Build history of the part. All positions in model axes, mm. A direction names the side the tool comes from. Give positions to 0.01 mm unless a question says otherwise; leave off trailing zeros. Loops run counter-clockwise (first coordinate to the right, second up) from the corner with the lowest first, then second, coordinate; pieces in that order, holes last. Notation, with made-up numbers: (40.25, 53.25) - (68.25, 53.25) arc R11 cw to (68.25, 67.25) - close; hole circle Ø9 at (1.5, 53.25). An arc over 180 degrees is marked (long way). Return JSON: item names as keys, results as strings. Group by question number.
1) 3-axis set-ups, long thin cutter, end or side, ignore diameter. For faces 1 (the face through (-21, 0, -12)), 2 (the face through (-3.365, 1.972, -12.206)): which of +Z, -Z, +X, -X, +Y, -Y reach the whole face in a straight line?
2) Slice it at A-A (x = -4). List the corners of the cut face in (y, z).
3) Mould opens along X. For faces 3 (the face through (-13, 2, 15)), 4 (the face through (5.93, -0.699, 12.785)), 5 (the face through (12, 2, -2)) say: released by +X, released by -X, zero draft, split by the parting line, or undercut.
4) Drop a flat-ended pin along its axis: pin 1 (2 mm diameter, centred on x = 3.5, z = 4, fed in from -Y). Give the stop position or say it passes through.
5) Slice it at D-D (x = -24). List the corners of the cut face in (y, z), and give its area (3 significant figures).
6) Drill centre lines: probe 1 along X at (y, z) = (-0.6, 10); probe 2 along Z at (x, y) = (-4, 1.2); probe 3 along X at (y, z) = (-0.5, -11). Where is each one in solid material? Low to high. Write a range as from..to.
Autodesk Inventor part; units mm, degrees
ref_plane "YZ Plane" through (0, 0, 0) normal (1, 0, 0) x (0, 1, 0)
ref_plane "XZ Plane" through (0, 0, 0) normal (0, 1, 0) x (-1, 0, 0)
ref_plane "XY Plane" through (0, 0, 0) normal (0, 0, 1) x (1, 0, 0)
sketch "スケッチ1" plane through (0, 0, 0) normal (0, 1, 0) x (-1, 0, 0)
  line L0 (26, 0) -> (0, 0)
  line L1 (0, 0) -> (0, -15)
  line L2 (0, -15) -> (26, -15)
  line L3 (26, -15) -> (26, 0)
  line L4 (36.4849, 5.9511) -> (26, -20)
  line L5 (26, -20) -> (0, -20)
  line L6 (0, -20) -> (-10.4849, 5.9511)
  arc A0 (36.4849, 5.9511) -> (-10.4849, 5.9511) centre (13, -20) ccw
  line L7 (0, 0) -> (26, -15)
  line L8 (0, -15) -> (26, 0)
  line L9 (4, -2.3077) -> (22, -2.3077)
  line L10 (22, -2.3077) -> (22, -12.6923)
  line L11 (22, -12.6923) -> (4, -12.6923)
  line L12 (4, -12.6923) -> (4, -2.3077)
  circle A1 centre (4, -2.3077) radius 0.8
  circle A2 centre (4, -12.6923) radius 0.8
  circle A3 centre (22, -2.3077) radius 0.8
  circle A4 centre (22, -12.6923) radius 0.8
  circle A5 centre (13, -7.5) radius 0.8
  line L13 (38, 15) -> (-12, 15)
  line L14 (-12, 15) -> (-12, -20)
  line L15 (-12, -20) -> (38, -20)
  line L16 (38, -20) -> (38, 15)
  point P0 (22.6929, -13.0921)
  point P1 (21.2, -12.6923)
  point P2 (13, 15)
  point P3 (13, -7.5)
  point P4 (13, 15)
  point P5 (0, -20)
  dimension "d0" = 26
  dimension "d1" = 15
  dimension "d4" = 22
  dimension "d5" = 22
  dimension "d6" = 5
  dimension "d7" = 35
  dimension "d23" = 4
  dimension "d24" = 1.6
  dimension "d25" = 1.6
  dimension "d26" = 1.6
  dimension "d27" = 1.6
  dimension "d32" = 1.6
  dimension "d54" = 50
  dimension "d55" = 35
extrude "押し出し1" add sketch "スケッチ1" along normal blind 4 contours L8 A3 L9 A1 L7 L0 | L3 L7 A4 L10 A3 L8 | L7 A1 L12 A2 L8 L1 | L2 L8 A2 L11 A4 L7 | A3 L10 L8 | L8 L9 A3 | A1 L9 L7 | L7 L12 A1 | L10 A3 L8 | L8 A3 L9 | A3 L8 A5 L7 A1 L9 | L9 A1 L7 | L7 A1 L12 | A1 L7 A5 L8 A2 L12 | L11 A2 L8 A5 L7 A4 | A3 L10 A4 L7 A5 L8 | A0 L13 L16 L15 L4 | L4 L5 L6 A0 | A0 L6 L15 L14 L13
sketch "スケッチ5" plane through (0, 0, 0) normal (0, -1, 0) x (1, 0, 0)
  line L0 (12, -20) -> (-38, -20)
  line L1 (12, 15) -> (12, -20)
  line L2 (-38, 15) -> (12, 15)
  line L3 (-38, -20) -> (-38, 15)
  circle A0 centre (-13, -7.5) radius 0.8
  circle A1 centre (-4, -12.6923) radius 0.8
  circle A2 centre (-22, -12.6923) radius 0.8
  circle A3 centre (-13, -7.5) radius 2.5
  circle A4 centre (-4, -12.6923) radius 2.5
  circle A5 centre (-22, -12.6923) radius 2.5
  line L4 (10, 12.5) -> (2, 12.5)
  line L5 (2, 12.5) -> (2, -17.5)
  line L6 (2, -17.5) -> (10, -17.5)
  line L7 (10, -17.5) -> (10, 12.5)
  line L8 (-28, 12.5) -> (-36, 12.5)
  line L9 (-36, 12.5) -> (-36, -17.5)
  line L10 (-36, -17.5) -> (-28, -17.5)
  line L11 (-28, -17.5) -> (-28, 12.5)
  point P0 (0, 0)
  point P1 (10, -2.5)
  point P2 (12, -2.5)
  point P3 (-28, -2.5)
  dimension "d56" = 5
  dimension "d57" = 5
  dimension "d58" = 5
  dimension "d61" = 8
  dimension "d62" = 30
  dimension "d63" = 2
  dimension "d64" = 2
extrude "押し出し5" add sketch "スケッチ5" along normal blind 1 contours L0 L3 L2 L1
fillet "フィレット3" radius 1 8 edges at (6, -1, 12.5) (10, -1, -2.5) (6, -1, -17.5) (2, -1, -2.5) (-28, -1, -2.5) (-32, -1, -17.5) (-36, -1, -2.5) (-32, -1, 12.5)
equation "\"d5\" = d4"
equation "\"BendRadius\" = Thickness"
equation "\"BendReliefWidth\" = Thickness"
equation "\"BendReliefDepth\" = 0.5 * Thickness"
equation "\"CornerReliefSize\" = 4 * Thickness"
equation "\"MinimumRemnant\" = 2 * Thickness"
equation "\"TransitionRadius\" = BendRadius"
equation "\"JacobiRadiusSize\" = BendRadius"
equation "\"GapSize\" = Thickness"
properties part number "toe_sole_front"
Results:
{
 "1": {"face 1": "-Y", "face 2": "+Y, -Y"},
 "2": {"outline": "(-1, -20) - (4, -20) - (4, -13.49) - (0, -13.49) - (0, -15.19) - (-1, -15.19) - close; (-1, -10.19) - (0, -10.19) - (0, -11.89) - (4, -11.89) - (4, 15) - (-1, 15) - close"},
 "3": {"face 3": "zero draft", "face 4": "undercut", "face 5": "released by +X"},
 "4": {"pin 1": "y = 0"},
 "5": {"outline": "(-1, -20) - (4, -20) - (4, 15) - (-1, 15) - (-1, -11.19) - (0, -11.19) - (0, -14.19) - (-1, -14.19) - close", "area": "172 mm2"},
 "6": {"probe 1": "-38..-36.2, -27.8..1.8, 10.2..12", "probe 2": "-20..-13.49, -11.89..15", "probe 3": "-38..-36.13, -27.87..-23.84, -20.16..-5.84, -2.16..1.87, 10.13..12"}
}
